Autodesk Fusion 360 part; units mm, degrees
sketch "Sketch1" plane through (0, 0, 0) normal (0, 1, 0) x (1, 0, 0)
  line L0 (5.5, 5.5) -> (-5.5, 5.5)
  line L1 (-5.5, 5.5) -> (-5.5, -5.5)
  line L2 (-5.5, -5.5) -> (5.5, -5.5)
  line L3 (5.5, -5.5) -> (5.5, 5.5)
  line L4 (5.5, 5.5) -> (-5.5, -5.5) construction
  line L5 (-5.5, 5.5) -> (5.5, -5.5) construction
  dimension "d1" = 11
  dimension "d2" = 11
extrude "Extrude1" add sketch "Sketch1" along normal blind 2
sketch "Sketch2" plane through (0, 2, 0) normal (0, 1, 0) x (-1, 0, 0)
  line L0 (-5.5, 5.5) -> (-5.5, -5.5)
  line L1 (-5.5, -5.5) -> (5.5, -5.5)
  line L2 (5.5, -5.5) -> (5.5, 5.5)
  line L3 (5.5, 5.5) -> (-5.5, 5.5)
  circle A0 centre (0, 0) radius 5.25
  dimension "d5" = 10.5
extrude "Extrude2" add sketch "Sketch2" along normal blind 7 contours A0
sketch "Sketch3" plane through (0, 9, 0) normal (0, 1, 0) x (-1, 0, 0)
  circle A0 centre (0, 0) radius 5.25
  line L0 (1.25, 5.25) -> (-1.25, 5.25)
  line L1 (-1.25, 5.25) -> (-1.25, -5.25)
  line L2 (-1.25, -5.25) -> (1.25, -5.25)
  line L3 (1.25, -5.25) -> (1.25, 5.25)
  line L4 (1.25, 5.25) -> (-1.25, -5.25) construction
  line L5 (-1.25, 5.25) -> (1.25, -5.25) construction
  dimension "d8" = 2.5
  dimension "d9" = 10.5
extrude "Extrude3" add sketch "Sketch3" along normal blind 3 contours A0 L1 L3
sketch "Sketch4" plane through (0, 0, 0) normal (0, -1, 0) x (1, 0, 0)
  line L0 (5.5, -5.5) -> (5.5, 5.5)
  line L1 (5.5, 5.5) -> (-5.5, 5.5)
  line L2 (-5.5, 5.5) -> (-5.5, -5.5)
  line L3 (-5.5, -5.5) -> (5.5, -5.5)
  line L4 (1.05, 1.55) -> (-1.05, 1.55)
  line L5 (-1.05, 1.55) -> (-1.05, -1.55)
  line L6 (-1.05, -1.55) -> (1.05, -1.55)
  line L7 (1.05, -1.55) -> (1.05, 1.55)
  line L8 (1.05, 1.55) -> (-1.05, -1.55) construction
  line L9 (-1.05, 1.55) -> (1.05, -1.55) construction
  dimension "d12" = 2.1
  dimension "d13" = 3.1
extrude "Extrude4" cut sketch "Sketch4" against normal blind 3 contours L4 L5 L6 L7
Check sheet for the modelled part. Datum: model origin and axes. Units: mm. A direction names the side the tool comes from. Coordinates: 2 decimals unless noted, no trailing zeros. Order: outer loops, then holes, each group sorted by start corner. A loop starts at its lowest first (then second) coordinate and runs counter-clockwise, first axis right, second up. Notation, with made-up numbers: M 27,-32 L 49,-32 A14 cw 49,-16 Z; hole C -28.5,56.25 d9. An arc over 180 degrees is marked long. One line per question, with ' | ' between items. Start each with the question number.
Item 1: Sectioned sample at A-A on x = 0. Record the cut outline in (y, z).
Item 2: Sectioned sample at D-D on y = 6.75. Record the cut outline in (x, z).
Item 3: Mould release check, pull along X, two halves, no side actions. Record for faces 1 (the flat face through (-3, 2, -5)), 2 (the cylindrical face through (5.245, 5.819, -0.231)), 3 (the flat face through (1.25, 10, 0)), 4 (the flat face through (-1.05, 1, 0)): pulls with the +X half, pulls with the -X half, needs draft (parallel to the pull), parting line crosses it, or undercut.
Item 4: Material ranges on line 1 (Y direction, x = -1.75, z = -0.75); line 2 (Y direction, x = -4.5, z = -3); line 3 (Z direction, x = -1, y = 1.75), recorded low to high.
Item 5: Gauge pin test, flat ends, axial feed: P1, Ø1.5, axis at x = 0.5, y = 9.5, coming from the -Z side; P2, Ø1.7, axis at x = -0.5, z = -0.5, coming from the -Y side; P3, Ø3, axis at x = 3, z = 0.5, coming from the +Y side; P4, Ø1.5, axis at x = 4, y = 8.5, coming from the +Z side. Record the tip position at first contact, or that the pin passes through.
Item 6: Access from +Z, -Z, +X, -X, +Y, -Y to the whole of each face (thin tool, end or side, straight path). Record for faces 5 (the flat face through (1.05, 1, 0)), 6 (the flat face through (-1.25, 10, 0)), 7 (the flat face through (0, 1, -5.5)), 8 (the flat face through (5.5, 1, 0)), 9 (the flat face through (3, 9, 0)).
Item 7: Sectioned sample at B-B on z = 0. Record the cut outline in (x, y), and give its area (3 significant figures).
Item 8: Sectioned sample at C-C on y = 2.75. Record the cut outline in (x, z), and give its area (3 significant figures).
Answer below:
1) outline: M 0,-5.5 L 2,-5.5 L 2,-5.25 L 12,-5.25 L 12,5.25 L 2,5.25 L 2,5.5 L 0,5.5 L 0,1.55 L 3,1.55 L 3,-1.55 L 0,-1.55 Z
2) outline: C 0,0 d10.5
3) face 1: needs draft | face 2: parting line crosses it | face 3: pulls with the +X half | face 4: undercut
4) line 1: y = 0 to 9 | line 2: y = 0 to 2 | line 3: z = -5.5 to -1.55, 1.55 to 5.5
5) P1: stops at z = -5.25 | P2: stops at y = 0 | P3: stops at y = 9 | P4: stops at z = 4.12
6) face 5: -Y | face 6: +Z, -Z, -X, +Y | face 7: -Z, +X, -X, +Y, -Y | face 8: +Z, -Z, +X, +Y, -Y | face 9: +Z, -Z, +X, +Y
7) outline: M -5.5,0 L -1.05,0 L -1.05,3 L 1.05,3 L 1.05,0 L 5.5,0 L 5.5,2 L 5.25,2 L 5.25,9 L 1.25,9 L 1.25,12 L -1.25,12 L -1.25,9 L -5.25,9 L -5.25,2 L -5.5,2 Z | area: 96.7 mm^2
8) outline: C 0,0 d10.5; hole M -1.05,-1.55 L 1.05,-1.55 L 1.05,1.55 L -1.05,1.55 Z | area: 80.1 mm^2
